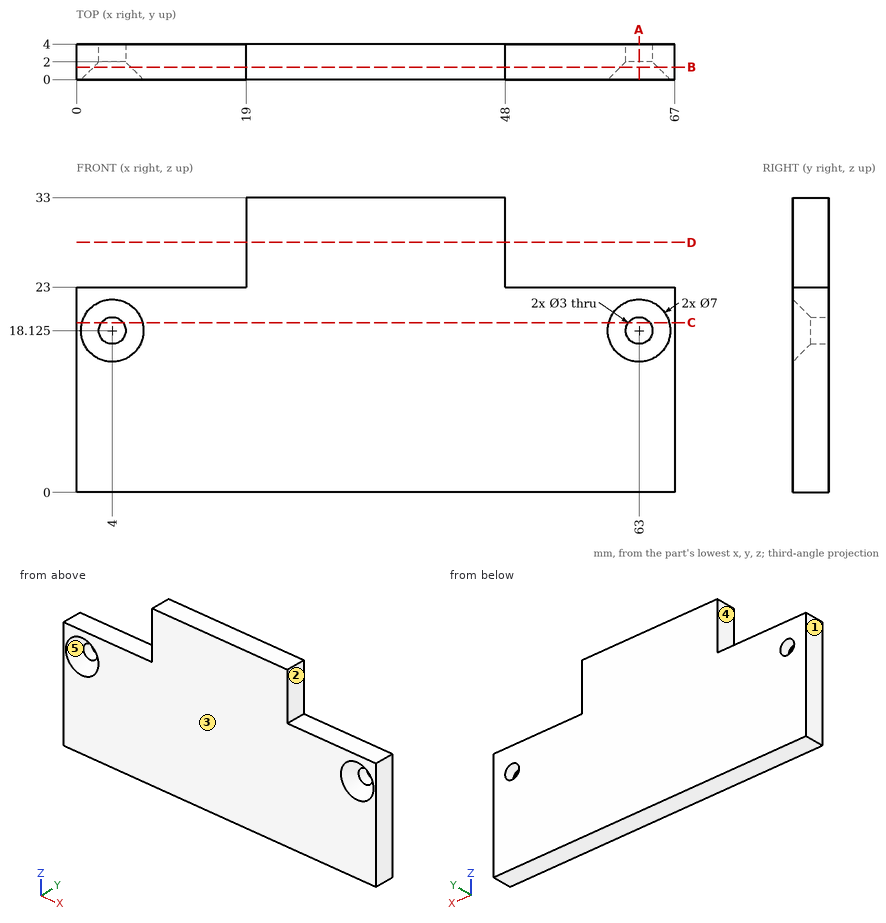
Answer from the drawing. Dimensions are ordinates in mm from the lowest x, y and z of the part. A direction names the side the tool comes from. Give positions to 0.01 mm unless a question says otherwise; leave off trailing zeros. Write each loop counter-clockwise with the first axis right and the second up, starting at its lowest first coordinate (ties: lowest second). Pieces come first, ordered by that corner, then holes. Notation, with made-up numbers: (-26, -22.5) - (1, -22.5) arc R22 cw to (1, -9.5) - close; hole circle Ø1 at (1, -22). An arc over 180 degrees is marked (long way). One line per item, written item: value. Start each with the question number.
1. Consider probe 1 along Z at (x, y) = (63, 2.95) (3 decimals); probe 2 along X at (y, z) = (3.75, 17.5); probe 3 along X at (y, z) = (0.55, 17.5). Determine where each line is inside the solid, lowest interval first.
2. Find section C-C (z = 19). State how many separate pieces and enclosed holes the cut face has, then the cut area to 3 significant figures.
3. Find section A-A (x = 63). Write down the section's boundary in (y, z) (3 decimals).
4. Given pin 1 (2.5 mm diameter, centred on x = 4, z = 18.125, fed in from +Y); pin 2 (2 mm diameter, centred on y = 1.5, z = 4.5, fed in from -X); pin 3 (2 mm diameter, centred on x = 9, y = 1.5, fed in from +Z); pin 4 (2 mm diameter, centred on y = 2.5, z = 30.5, fed in from -X), each flat-ended and moving along its own axis, determine where each tip first touches the part or whether it passes through.
5. Find section D-D (z = 28). Write down the section's boundary in (x, y), then the cut area to 3 significant figures.
6. For the marked faces 1 and 2, determine the directions among +Z, -Z, +X, -X, +Y, -Y from which every point of the face is accessible in a straight line to the end or side of a thin tool.
7. Find section B-B (y = 1.4). Write down the section's boundary in (x, z) (3 decimals).
8. For a pull along X with two mould halves and no side action, classify the marked faces 3, 4 and 5 as +X half, -X half, draft (parallel to the pull), parting line (faces both ways), or undercut.
Geometry results:
1. probe 1: 0 to 16.625, 19.625 to 23
1. probe 2: 0 to 2.64, 5.36 to 61.64, 64.36 to 67
1. probe 3: 0 to 1.12, 6.88 to 60.12, 65.88 to 67
2. separate pieces: 3
2. enclosed holes: 0
2. area: 240 mm2
3. outline: (0, 0) - (4, 0) - (4, 16.625) - (2, 16.625) - (0, 14.625) - close; (0, 21.625) - (2, 19.625) - (4, 19.625) - (4, 23) - (0, 23) - close
4. pin 1: through
4. pin 2: x = 0
4. pin 3: z = 23
4. pin 4: x = 19
5. outline: (19, 0) - (48, 0) - (48, 4) - (19, 4) - close
5. area: 116 mm2
6. face 1: +Z, -Z, -X, +Y, -Y
6. face 2: +Z, +X, +Y, -Y
7. outline: (0, 0) - (67, 0) - (67, 23) - (48, 23) - (48, 33) - (19, 33) - (19, 23) - (0, 23) - close; hole circle Ø4.2 at (4, 18.125); hole circle Ø4.2 at (63, 18.125)
8. face 3: draft
8. face 4: -X half
8. face 5: undercut
